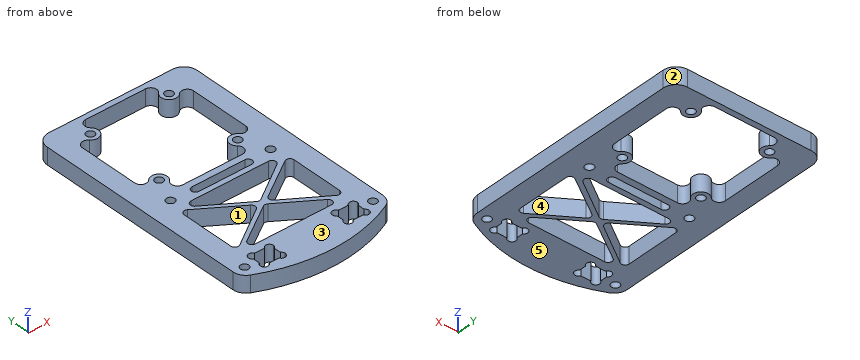
from build123d import *

# Parameters (mm, degrees)
F0_R     = 1.55
F0_W     = 8
F0_H     = 6.35
F0_R_2   = 1.6
F1_DEPTH = 6.35
F3_DEPTH = 25
F4_R     = 1.5
F6_DEPTH = 25


with BuildPart() as f1:
    # F0 (on Top) → F1 (new body)
    with BuildSketch(Plane.XY):
        with BuildLine():
            ThreePointArc((28.575, 42.02), (27.1105339059, 45.5555339059), (23.575, 47.02))
            Line((23.575, 47.02), (-23.575, 47.02))
            ThreePointArc((-23.575, 47.02), (-27.1105339059, 45.5555339059), (-28.575, 42.02))
            Line((-28.575, 42.02), (-28.575, -39.0813798373))
            ThreePointArc((-28.575, -39.0813798373), (-27.8126666433, -41.7350907147), (-25.7581274318, -43.5795966636))
            ThreePointArc((-25.7581274318, -43.5795966636), (0, -49.5), (25.7581274318, -43.5795966636))
            ThreePointArc((25.7581274318, -43.5795966636), (27.8126666433, -41.7350907147), (28.575, -39.0813798373))
            Line((28.575, -39.0813798373), (28.575, 42.02))
        make_face()
        with Locations((-24.5, -39.5)):
            Circle(F0_R, mode=Mode.SUBTRACT)
        with Locations((-16, -39.5)):
            Rectangle(F0_W, F0_H, mode=Mode.SUBTRACT)
        with Locations((16, -39.5)):
            Rectangle(F0_W, F0_H, mode=Mode.SUBTRACT)
        with Locations((24.5, -39.5)):
            Circle(F0_R, mode=Mode.SUBTRACT)
        with BuildLine():
            ThreePointArc((10.075, 0), (11.575, -1.5), (10.075, -3))
            Line((10.075, -3), (0, -3))
            Line((0, -3), (-10.075, -3))
            ThreePointArc((-10.075, -3), (-11.575, -1.5), (-10.075, 0))
            Line((-10.075, 0), (0, 0))
            Line((0, 0), (10.075, 0))
        make_face(mode=Mode.SUBTRACT)
        with Locations((-19.075, -0.98)):
            Circle(F0_R_2, mode=Mode.SUBTRACT)
        with Locations((-15, 8.7)):
            Circle(F0_R, mode=Mode.SUBTRACT)
        with Locations((-15, 38.7)):
            Circle(F0_R, mode=Mode.SUBTRACT)
        with Locations((19.075, -0.98)):
            Circle(F0_R_2, mode=Mode.SUBTRACT)
        with Locations((15, 8.7)):
            Circle(F0_R, mode=Mode.SUBTRACT)
        with BuildLine():
            Line((-11.411128311, 44.9), (0, 44.9))
            Line((0, 44.9), (11.411128311, 44.9))
            ThreePointArc((11.411128311, 44.9), (13.5538650552, 43.435870352), (12.9685631949, 40.9075471698))
            ThreePointArc((12.9685631949, 40.9075471698), (12.8786796564, 36.5786796564), (17.2075471698, 36.6685631949))
            ThreePointArc((17.2075471698, 36.6685631949), (19.735870352, 37.2538650552), (21.2, 35.111128311))
            Line((21.2, 35.111128311), (21.2, 23.7))
            Line((21.2, 23.7), (21.2, 12.288871689))
            ThreePointArc((21.2, 12.288871689), (19.735870352, 10.1461349448), (17.2075471698, 10.7314368051))
            ThreePointArc((17.2075471698, 10.7314368051), (12.8786796564, 10.8213203436), (12.9685631949, 6.4924528302))
            ThreePointArc((12.9685631949, 6.4924528302), (13.5538650552, 3.964129648), (11.411128311, 2.5))
            Line((11.411128311, 2.5), (0, 2.5))
            Line((0, 2.5), (-11.411128311, 2.5))
            ThreePointArc((-11.411128311, 2.5), (-13.5538650552, 3.964129648), (-12.9685631949, 6.4924528302))
            ThreePointArc((-12.9685631949, 6.4924528302), (-12.8786796564, 10.8213203436), (-17.2075471698, 10.7314368051))
            ThreePointArc((-17.2075471698, 10.7314368051), (-19.735870352, 10.1461349448), (-21.2, 12.288871689))
            Line((-21.2, 12.288871689), (-21.2, 23.7))
            Line((-21.2, 23.7), (-21.2, 35.111128311))
            ThreePointArc((-21.2, 35.111128311), (-19.735870352, 37.2538650552), (-17.2075471698, 36.6685631949))
            ThreePointArc((-17.2075471698, 36.6685631949), (-12.8786796564, 36.5786796564), (-12.9685631949, 40.9075471698))
            ThreePointArc((-12.9685631949, 40.9075471698), (-13.5538650552, 43.435870352), (-11.411128311, 44.9))
        make_face(mode=Mode.SUBTRACT)
        with Locations((15, 38.7)):
            Circle(F0_R, mode=Mode.SUBTRACT)
    extrude(amount=F1_DEPTH)

    # F2 (on face) → F3 (cut)
    with BuildSketch(Plane.XY.offset(6.35)):
        Polygon((-20.75, -32), (-1.3711180124, -19.0807453416), (-20.75, -6), align=None)
        Polygon((0, -18.1666666667), (19.75, -5), (-19.75, -5), align=None)
        Polygon((20.75, -32), (20.75, -6.5), (1.4462616822, -19.1308411215), align=None)
        Polygon((19.25, -33), (0.0533433945, -20.0422567913), (-19.75, -33), align=None)
    extrude(amount=-F3_DEPTH, mode=Mode.SUBTRACT)

    # F4
    f4_edges = [f1.edges().sort_by_distance(p)[0] for p in [
        (-20.75, -6, 3.175),
        (-20.75, -32, 3.175),
        (-19.75, -5, 3.175),
        (19.75, -5, 3.175),
        (20.75, -6.5, 3.175),
        (20.75, -32, 3.175),
        (19.25, -33, 3.175),
        (-19.75, -33, 3.175),
        (0.053343, -20.042257, 3.175),
        (1.446262, -19.130841, 3.175),
        (0, -18.166667, 3.175),
        (-1.371118, -19.080745, 3.175),
    ]]
    fillet(f4_edges, radius=F4_R)

    # F5 (on face) → F6 (cut)
    with BuildSketch(Plane(origin=(0, 0, 0), x_dir=(1, 0, 0), z_dir=(0, 0, -1))):
        with BuildLine():
            Line((-12, 36.325), (-14.1268090018, 36.325))
            ThreePointArc((-14.1268090018, 36.325), (-12.4460374222, 35.4514330797), (-11.25, 36.9203125))
            ThreePointArc((-11.25, 36.9203125), (-11.4509618943, 37.6703125), (-12, 38.2193506057))
            Line((-12, 38.2193506057), (-12, 36.325))
        make_face()
        with BuildLine():
            ThreePointArc((-11.25, 42.0796875), (-12.4460374222, 43.5485669203), (-14.1268090018, 42.675))
            Line((-14.1268090018, 42.675), (-12, 42.675))
            Line((-12, 42.675), (-12, 40.7806493943))
            ThreePointArc((-12, 40.7806493943), (-11.4509618943, 41.3296875), (-11.25, 42.0796875))
        make_face()
        with BuildLine():
            ThreePointArc((-17.8731909982, 42.675), (-20.2476790243, 43.1997931042), (-20, 40.7806493943))
            Line((-20, 40.7806493943), (-20, 42.675))
            Line((-20, 42.675), (-17.8731909982, 42.675))
        make_face()
        with BuildLine():
            Line((-20, 36.325), (-20, 38.2193506057))
            ThreePointArc((-20, 38.2193506057), (-20.2476790243, 35.8002068958), (-17.8731909982, 36.325))
            Line((-17.8731909982, 36.325), (-20, 36.325))
        make_face()
        with BuildLine():
            Line((12, 36.325), (12, 38.2193506057))
            ThreePointArc((12, 38.2193506057), (11.7523209757, 35.8002068958), (14.1268090018, 36.325))
            Line((14.1268090018, 36.325), (12, 36.325))
        make_face()
        with BuildLine():
            ThreePointArc((14.1268090018, 42.675), (11.7523209757, 43.1997931042), (12, 40.7806493943))
            Line((12, 40.7806493943), (12, 42.675))
            Line((12, 42.675), (14.1268090018, 42.675))
        make_face()
        with BuildLine():
            ThreePointArc((20.75, 42.0796875), (19.5539625778, 43.5485669203), (17.8731909982, 42.675))
            Line((17.8731909982, 42.675), (20, 42.675))
            Line((20, 42.675), (20, 40.7806493943))
            ThreePointArc((20, 40.7806493943), (20.5490381057, 41.3296875), (20.75, 42.0796875))
        make_face()
        with BuildLine():
            Line((20, 36.325), (17.8731909982, 36.325))
            ThreePointArc((17.8731909982, 36.325), (19.5539625778, 35.4514330797), (20.75, 36.9203125))
            ThreePointArc((20.75, 36.9203125), (20.5490381057, 37.6703125), (20, 38.2193506057))
            Line((20, 38.2193506057), (20, 36.325))
        make_face()
    extrude(amount=-F6_DEPTH, mode=Mode.SUBTRACT)


solid = f1.part
Could you check a few things on this model? Use its own coordinates, in mm. Face numbers are marked on the shaded views. A direction names the side the tool comes from. Give positions to 0.01 mm unless a question says otherwise; leave off trailing zeros. Order: outer loops, then holes, each group sorted by start corner. A loop starts at its lowest first (then second) coordinate and runs counter-clockwise, first axis right, second up. Notation, with made-up numbers: (36, -3) - (53, -3) arc R9 ccw to (53, 2) - close; hole circle Ø7 at (-36.5, -9). An arc over 180 degrees is marked (long way). One line per question, with ' | ' between items. Start each with the question number.
Item 1: For the marked faces 4 and 5, which set-ups out of +Z, -Z, +X, -X, +Y, -Y let a thin tool reach every point of the face, with its end or its side?
Item 2: I want a section at D-D on z = 3.5. Give the number of separate pieces and of enclosed holes in the cut face, then the cut area to 3 significant figures.
Item 3: I want a section at C-C on y = -0.98. Write out the boundary of the cut face in (x, z) (3 decimals), then the cut area to 3 significant figures.
Item 4: I need wall thicknesses on probe 1 along X at (y, z) = (-19, 5) (3 decimals); probe 2 along X at (y, z) = (19, 5.5) (3 decimals); probe 3 along X at (y, z) = (9, 5.5) (3 decimals). Which ranges of each line are inside material? Lowest first, please. Write a range as [from, to].
Item 5: I want a section at A-A on y = 15. Write out the boundary of the cut face in (x, z) (3 decimals), then the cut area to 3 significant figures.
Item 6: Thinking about a two-plate mould opening in Y: for the marked faces 1, 2 and 3, which applies, pulls with the +Y half, pulls with the -Y half, needs draft (parallel to the pull), parting line crosses it, or undercut?
Item 7: I'm going to push flat-ended pins straight in: pin 1 Ø3 at (x, y) = (15, 38.7) entering from -Z; pin 2 Ø3 at (x, z) = (-0.5, 1.5) entering from -Y. Where does each tip first touch, or does it pass through?
Verdict:
1) face 4: +Z, -Z | face 5: -Z, +X, -X, +Y, -Y
2) separate pieces: 1 | enclosed holes: 16 | area: 2,610 mm^2
3) outline: (-28.575, 0) - (-20.675, 0) - (-20.675, 6.35) - (-28.575, 6.35) - close; (-17.475, 0) - (-11.482, 0) - (-11.482, 6.35) - (-17.475, 6.35) - close; (11.482, 0) - (17.475, 0) - (17.475, 6.35) - (11.482, 6.35) - close; (20.675, 0) - (28.575, 0) - (28.575, 6.35) - (20.675, 6.35) - close | area: 176 mm^2
4) probe 1: [-28.575, -20.75], [-2.565, 2.675], [20.75, 28.575] | probe 2: [-28.575, -21.2], [21.2, 28.575] | probe 3: [-28.575, -16.521], [-13.479, -12.015], [12.015, 13.479], [16.521, 28.575]
5) outline: (-28.575, 0) - (-21.2, 0) - (-21.2, 6.35) - (-28.575, 6.35) - close; (21.2, 0) - (28.575, 0) - (28.575, 6.35) - (21.2, 6.35) - close | area: 93.7 mm^2
6) face 1: undercut | face 2: pulls with the +Y half | face 3: needs draft
7) pin 1: through | pin 2: y = -49.5
